Part model, mm, in its own coordinate system. Round coordinates to 2 decimals unless told otherwise and drop trailing zeros. Loops run counter-clockwise (first coordinate to the right, second up) from the corner with the lowest first, then second, coordinate; pieces in that order, holes last. Notation, with made-up numbers: (38.25, -39) - (78.25, -39) arc R29 cw to (78.25, -6) - close; hole circle Ø11 at (62.25, 24.5). An arc over 180 degrees is marked (long way). Write each question's results on one line, items separated by ' | '. Start each with the question number.
(1) Cut at D-D, the plane y = -7. List the corners of the cut face in (x, z) (3 decimals).
(2) Mould opens along X. For faces 1 (the face through (76.29, 117.77, 1.61)), 2 (the face through (-7.58, 54.85, 1.57)), 3 (the face through (0.279, -25.397, 1.565)), 4 (the face through (33, 80, 0)) say: released by +X, released by -X, zero draft, split by the parting line, or undercut.
(3) Cut at B-B, the plane x = 0. List the corners of the cut face in (y, z) (1 decimal), then the cut area to 3 significant figures.
(4) Flat gauge pins, fed straight in: P1, Ø3.5, axis at x = 54.67, y = 157.22, coming from the +Z side; P2, Ø1, axis at y = 56.5, z = 2, coming from the -X side; P3, Ø1.5, axis at x = 47.5, z = 1.5, coming from the -Y side. Where does each tip first touch, or does it go through?
(5) Drill centre lines: L1, parallel to Y at x = 0, z = 1.3; L2, parallel to X at y = -12.7, z = 1.7; L3, parallel to X at y = 21.5, z = 1.9. Where is each one in solid material? Low to high.
(6) Cut at A-A, the plane y = 12.7. List the corners of the cut face in (x, z) (1 decimal).
(7) Cut at C-C, the plane z = 2.45. Give the number of separate pieces and of enclosed holes in the cut face, then the cut area to 3 significant figures.
Autodesk Inventor part; units mm, degrees
ref_plane "YZ Plane" through (0, 0, 0) normal (1, 0, 0) x (0, 1, 0)
ref_plane "XZ Plane" through (0, 0, 0) normal (0, 1, 0) x (-1, 0, 0)
ref_plane "XY Plane" through (0, 0, 0) normal (0, 0, 1) x (1, 0, 0)
sketch "Sketch1" plane through (0, 0, 0) normal (0, 0, 1) x (1, 0, 0)
  line L0 (-12.7, 25.4) -> (12.7, 25.4)
  line L1 (12.7, 25.4) -> (12.7, -25.4)
  line L2 (12.7, -25.4) -> (-12.7, -25.4)
  line L3 (-12.7, -25.4) -> (-12.7, 25.4)
  line L4 (-12.7, 25.4) -> (12.7, -25.4) construction
  line L5 (12.7, 25.4) -> (-12.7, -25.4) construction
  line L6 (72.5658, 158.7842) -> (111.4809, 126.1305)
  line L7 (111.4809, 126.1305) -> (95.1541, 106.673)
  line L8 (95.1541, 106.673) -> (56.239, 139.3266)
  line L9 (56.239, 139.3266) -> (72.5658, 158.7842)
  line L10 (72.5658, 158.7842) -> (95.1541, 106.673) construction
  line L11 (111.4809, 126.1305) -> (56.239, 139.3266) construction
  line L12 (74.1312, 140.892) -> (93.5887, 124.5652) construction
  line L13 (0, -12.7) -> (0, 12.7) construction
  line L14 (-12.7, -25.4) -> (12.7, -25.4)
  line L15 (12.7, -25.4) -> (12.7, -50.8)
  line L16 (12.7, -50.8) -> (-12.7, -50.8)
  line L17 (-12.7, -50.8) -> (-12.7, -25.4)
  circle A0 centre (0, -38.1) radius 12.7
  line L18 (75.6966, 122.9998) -> (56.239, 139.3266)
  line L19 (56.239, 139.3266) -> (-17.8482, 51.033)
  line L20 (-17.8482, 51.033) -> (1.6094, 34.7061)
  line L21 (1.6094, 34.7061) -> (75.6966, 122.9998)
  line L22 (72.5658, 158.7842) -> (56.239, 139.3266)
  line L23 (56.239, 139.3266) -> (36.7815, 155.6534)
  line L24 (36.7815, 155.6534) -> (53.1083, 175.111)
  line L25 (53.1083, 175.111) -> (72.5658, 158.7842)
  line L26 (54.6737, 157.2188) -> (74.1312, 140.892) construction
  arc A1 (62.8371, 166.9476) -> (46.5103, 147.49) centre (54.6737, 157.2188) ccw
  circle A2 centre (93.5887, 124.5652) radius 12.7
  line L27 (192.4417, 25.039) -> (17.324, 171.9802)
  circle A3 centre (0, -12.7) radius 12.7
  arc A4 (7.7203, 81.5042) -> (-12.7, 25.4) centre (74.5827, 25.4) ccw
  arc A5 (27.1778, 65.1774) -> (12.7, 25.4) centre (74.5827, 25.4) ccw
  point P0 (0, 0)
  point P1 (0, 0)
  point P2 (0, 0)
  point P3 (83.86, 132.7286)
  point P4 (83.86, 132.7286)
  point P5 (-12.7, -38.1)
  point P6 (12.7, -38.1)
  point P7 (-12.7, -4.4935)
  point P8 (12.7, -4.4935)
  point P9 (75.6966, 122.9998)
  point P10 (85.4253, 114.8364)
  point P11 (101.7521, 134.294)
  point P12 (-12.7, -12.7)
  point P13 (12.7, -12.7)
  dimension "d0" = 25.4
  dimension "d1" = 50.8
  dimension "d2" = 25.4
  dimension "d3" = 12.7
  dimension "d17" = 127
extrude "Extrusion1" add sketch "Sketch1" along normal blind 3.175 contours A4 L20 L21 A5 L0 | L0 L1 A3 L3 | A3 | A4 L19 L8 L21 L20 | L8 L9 L6 A2 | L23 A1 L25 L9 | A2
hole "Hole1" at (0, -12.7, 0) at (0, 12.7, 0) at (93.5887, 124.5652, 0) at (74.1312, 140.892, 0) at (0, -38.1, 0) at (54.6737, 157.2188, 0) direction (0, 0, 1) diameter 4.445 end through all
fillet "Fillet1" radius 12.7 2 edges at (56.239, 139.3266, 1.5875) (75.6966, 122.9998, 1.5875)
properties part number "Hood Upper Bracket" material "PET Plastic"
A:
1) outline: (-12.7, 0) - (12.7, 0) - (12.7, 3.175) - (-12.7, 3.175) - close
2) face 1: undercut | face 2: released by -X | face 3: split by the parting line | face 4: zero draft
3) outline: (-25.4, 0) - (-14.9, 0) - (-14.9, 3.2) - (-25.4, 3.2) - close; (-10.5, 0) - (10.5, 0) - (10.5, 3.2) - (-10.5, 3.2) - close; (14.9, 0) - (70.7, 0) - (70.7, 3.2) - (14.9, 3.2) - close | area: 277 mm2
4) P1: through | P2: x = -7.16 | P3: y = 88.5
5) L1: -25.4 to -14.92, -10.48 to 10.48, 14.92 to 70.74 | L2: -12.7 to -2.22, 2.22 to 12.7 | L3: -12.7 to 12.7
6) outline: (-12.7, 0) - (-2.2, 0) - (-2.2, 3.2) - (-12.7, 3.2) - close; (2.2, 0) - (12.7, 0) - (12.7, 3.2) - (2.2, 3.2) - close
7) separate pieces: 1 | enclosed holes: 5 | area: 6,250 mm2
